from build123d import *

# Parameters (mm, degrees)
F1_DEPTH = 50.8
F2_R     = 11.1125
F3_W     = 20.6375
F3_H     = 29.0905938273
F3_H_2   = 50.5422030863
F4_DEPTH = 33.3385
F5_SIZE  = 4.7625


with BuildPart() as f1:
    # F0 (on Right) → F1 (new body, symmetric)
    with BuildSketch(Plane.YZ):
        with BuildLine():
            Line((-63.5, 4.7625), (-63.5, 0))
            Line((-63.5, 0), (-6.35, 0))
            Line((-6.35, 0), (7.3786968916, 25.2575142941))
            ThreePointArc((7.3786968916, 25.2575142941), (9.7123359116, 27.6829742473), (12.9577969137, 28.575))
            Line((12.9577969137, 28.575), (63.5, 28.575))
            Line((63.5, 28.575), (63.5, 33.3375))
            Line((63.5, 33.3375), (6.35, 33.3375))
            Line((6.35, 33.3375), (-7.3786968916, 8.0799857059))
            ThreePointArc((-7.3786968916, 8.0799857059), (-9.7123359116, 5.6545257527), (-12.9577969137, 4.7625))
            Line((-12.9577969137, 4.7625), (-63.5, 4.7625))
        make_face()
    extrude(amount=F1_DEPTH, both=True)

    # F2
    f2_edges = [f1.edges().sort_by_distance(p)[0] for p in [
        (0, 6.35, 33.3375),
        (0, -6.35, 0),
    ]]
    fillet(f2_edges, radius=F2_R)

    # F3 (on face) → F4 (cut, through all)
    with BuildSketch(Plane.XY.offset(33.3375)):
        with BuildLine():
            Line((-38.1, -36.5125), (-38.1, -46.0375))
            ThreePointArc((-38.1, -46.0375), (-30.1625, -53.975), (-22.225, -46.0375))
            Line((-22.225, -46.0375), (-22.225, -36.5125))
            ThreePointArc((-22.225, -36.5125), (-30.1625, -28.575), (-38.1, -36.5125))
        make_face()
        with BuildLine():
            ThreePointArc((38.1, -36.5125), (30.1625, -28.575), (22.225, -36.5125))
            Line((22.225, -36.5125), (22.225, -46.0375))
            ThreePointArc((22.225, -46.0375), (30.1625, -53.975), (38.1, -46.0375))
            Line((38.1, -46.0375), (38.1, -36.5125))
        make_face()
        with Locations((-40.48125, -1.5875)):
            Rectangle(F3_W, F3_H)
        with Locations((40.48125, -1.5875)):
            Rectangle(F3_W, F3_H)
        with BuildLine():
            ThreePointArc((9.525, 38.1), (0, 47.625), (-9.525, 38.1))
            ThreePointArc((-9.525, 38.1), (0, 28.575), (9.525, 38.1))
        make_face()
        with BuildLine():
            Line((9.525, 63.5), (-9.525, 63.5))
            Line((-9.525, 63.5), (-9.525, 38.1))
            ThreePointArc((-9.525, 38.1), (0, 47.625), (9.525, 38.1))
            Line((9.525, 38.1), (9.525, 63.5))
        make_face()
        with Locations((-40.48125, 38.2288984568)):
            Rectangle(F3_W, F3_H_2)
        with Locations((40.48125, 38.2288984568)):
            Rectangle(F3_W, F3_H_2)
    extrude(amount=-F4_DEPTH, mode=Mode.SUBTRACT)

    # F5
    f5_edges = [f1.edges().sort_by_distance(p)[0] for p in [
        (50.8, -63.5, 2.38125),
        (50.8, -16.132797, 2.38125),
        (-50.8, -63.5, 2.38125),
        (-50.8, -16.132797, 2.38125),
        (30.1625, 63.5, 30.95625),
        (-30.1625, 63.5, 30.95625),
        (9.525, 63.5, 30.95625),
        (-9.525, 63.5, 30.95625),
    ]]
    chamfer(f5_edges, length=F5_SIZE)


solid = f1.part
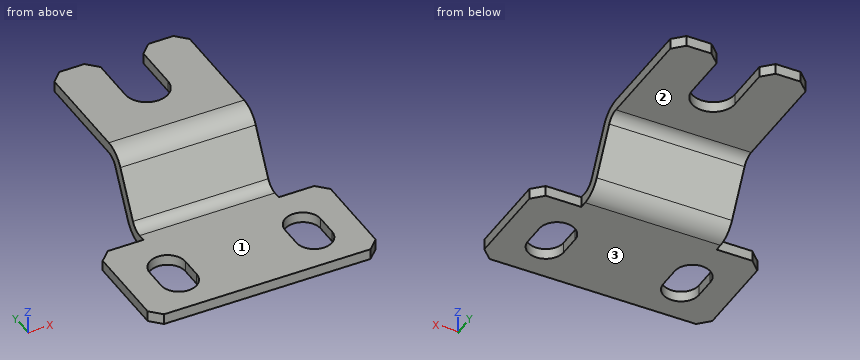
Model file for the job. Use its own axes, mm. Face numbers are marked on the shaded views. A direction names the side the tool comes from. Coordinates: 2 decimals unless noted, no trailing zeros. Order: outer loops, then holes, each group sorted by start corner. A loop starts at its lowest first (then second) coordinate and runs counter-clockwise, first axis right, second up. Notation, with made-up numbers: (61.25, 86.5) -> (99.25, 86.5) arc R16 ccw to (99.25, 108.5) -> close; hole circle Ø3 at (-8, -35.5). An arc over 180 degrees is marked (long way). Return JSON: item names as keys, results as strings. Group by question number.
Item 1: Saw through at D-D on y = 16.5. Write the cut outline in (x, z) (1 decimal), then the cut area to 3 significant figures.
Item 2: Wall check: line 1 along Z through (x, y) = (-29, 36.5) (1 decimal); line 2 along X through (y, z) = (-50.5, 1); line 3 along X through (y, z) = (34, 30.5). Give the ranges that are in metal, low to high. Write a range as [from, to].
Item 3: Saw through at C-C on z = 20. Write the cut outline in (x, y).
Item 4: Saw through at B-B on y = 45. Write the cut outline in (x, z) (1 decimal), then the cut area to 3 significant figures.
Item 5: Tool access for the marked faces 1, 2 and 3: list every direction of +Z, -Z, +X, -X, +Y, -Y with a clear straight run to the whole face (end or side of a thin tool).
Item 6: Flat gauge pins, fed straight in: P1, Ø15, axis at x = -10, y = -35.5, coming from the +Z side; P2, Ø5, axis at y = 52.5, z = 32, coming from the +X side; P3, Ø15, axis at x = 14, y = 42, coming from the -Z side (3 decimals). Where does each tip first touch, or does it go through?
Values found:
{
 "1": {"outline": "(-30.2, 28.6) -> (30.2, 28.6) -> (30.2, 33.3) -> (-30.2, 33.3) -> close", "area": "287 mm2"},
 "2": {"line 1": "z = [28.6, 33.3]", "line 2": "x = [-50.8, -36.73], [-23.6, 23.6], [36.73, 50.8]", "line 3": "x = [-30.16, -8.6], [8.6, 30.16]"},
 "3": {"outline": "(-30.16, -0.9) -> (30.16, -0.9) -> (30.16, 4.52) -> (-30.16, 4.52) -> close"},
 "4": {"outline": "(-30.2, 28.6) -> (-9.5, 28.6) -> (-9.5, 33.3) -> (-30.2, 33.3) -> close; (9.5, 28.6) -> (30.2, 28.6) -> (30.2, 33.3) -> (9.5, 33.3) -> close", "area": "197 mm2"},
 "5": {"face 1": "+Z, +X, -X, -Y", "face 2": "-Z, +X, -X, +Y", "face 3": "-Z, +X, -X, +Y, -Y"},
 "6": {"P1": "stops at z = 4.76", "P2": "stops at x = 30.16", "P3": "stops at z = 28.575"}
}
